Here's how the part is built. I have some questions about the finished solid (model axes, mm). Round coordinates to 2 decimals unless told otherwise and drop trailing zeros. Loops run counter-clockwise (first coordinate to the right, second up) from the corner with the lowest first, then second, coordinate; pieces in that order, holes last. Notation, with made-up numbers: M 83.25,18.25 L 117.25,18.25 A26 cw 117.25,40.25 Z; hole C -6.75,-25 d1. An arc over 180 degrees is marked long. Answer as a JSON object with one key per item and string values.
from build123d import *

# Parameters (mm, degrees)
SKETCH1_W           = 49
SKETCH1_H           = 33
SKETCH1_R           = 1.6
BOSS_EXTRUDE2_DEPTH = 3
FILLET1_R           = 2
SKETCH2_W           = 20
SKETCH2_H           = 27
CUT_EXTRUDE1_DEPTH  = 10


with BuildPart() as part:
    # Sketch1 → Boss-Extrude2 (new body)
    with BuildSketch(Plane.XY):
        with Locations((5.332147937, -0.241820768)):
            Rectangle(SKETCH1_W, SKETCH1_H)
        with Locations((-9.667852063, 9.758179232)):
            Circle(SKETCH1_R, mode=Mode.SUBTRACT)
        with Locations((20.332147937, 9.758179232)):
            Circle(SKETCH1_R, mode=Mode.SUBTRACT)
        with Locations((-9.667852063, -10.241820768)):
            Circle(SKETCH1_R, mode=Mode.SUBTRACT)
        with Locations((20.332147937, -10.241820768)):
            Circle(SKETCH1_R, mode=Mode.SUBTRACT)
    extrude(amount=BOSS_EXTRUDE2_DEPTH)

    # Fillet1
    fillet1_edges = [part.edges().sort_by_distance(p)[0] for p in [
        (-19.167852063, 16.258179232, 1.5),
        (29.832147937, 16.258179232, 1.5),
        (29.832147937, -16.741820768, 1.5),
        (-19.167852063, -16.741820768, 1.5),
    ]]
    fillet(fillet1_edges, radius=FILLET1_R)

    # Sketch2 → Cut-Extrude1 (cut)
    with BuildSketch(Plane.XY.offset(3)):
        with Locations((7.832147937, -0.241820768)):
            Rectangle(SKETCH2_W, SKETCH2_H)
    extrude(amount=-CUT_EXTRUDE1_DEPTH, mode=Mode.SUBTRACT)


solid = part.part
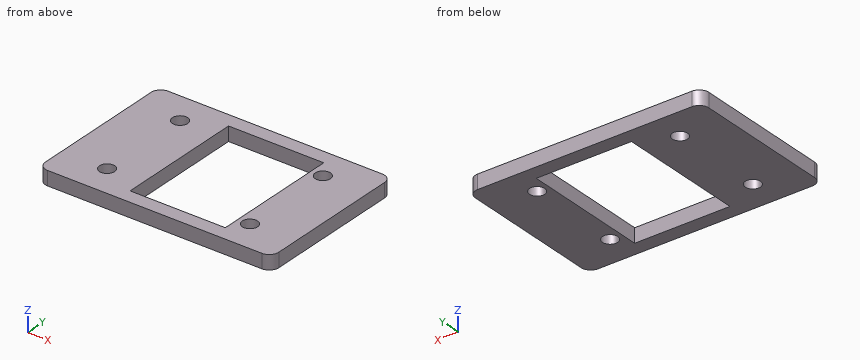
Item 1: I want a section at B-B, the plane y = -8. Please give me the cut outline in (x, z), then the cut area to 3 significant figures.
Resolved:
{"outline": "M -19.17,0 L -2.17,0 L -2.17,3 L -19.17,3 Z; M 17.83,0 L 29.83,0 L 29.83,3 L 17.83,3 Z", "area": "87.0 mm²"}
Item 2: I want a section at A-A, the plane x = -1.5. Please give me the cut outline in (y, z), then the cut area to 3 significant figures.
Resolved:
{"outline": "M -16.74,0 L -13.74,0 L -13.74,3 L -16.74,3 Z; M 13.26,0 L 16.26,0 L 16.26,3 L 13.26,3 Z", "area": "18.0 mm²"}
Item 3: I want a section at C-C, the plane y = 10.5. Please give me the cut outline in (x, z).
Resolved:
{"outline": "M -19.17,0 L -11.09,0 L -11.09,3 L -19.17,3 Z; M -8.25,0 L -2.17,0 L -2.17,3 L -8.25,3 Z; M 17.83,0 L 18.91,0 L 18.91,3 L 17.83,3 Z; M 21.75,0 L 29.83,0 L 29.83,3 L 21.75,3 Z"}
Item 4: I want a section at D-D, the plane z = 1.3. Please give me the cut outline in (x, y).
Resolved:
{"outline": "M -19.17,-14.74 A2 ccw -17.17,-16.74 L 27.83,-16.74 A2 ccw 29.83,-14.74 L 29.83,14.26 A2 ccw 27.83,16.26 L -17.17,16.26 A2 ccw -19.17,14.26 Z; hole C -9.67,-10.24 d3.2; hole C -9.67,9.76 d3.2; hole M -2.17,-13.74 L 17.83,-13.74 L 17.83,13.26 L -2.17,13.26 Z; hole C 20.33,-10.24 d3.2; hole C 20.33,9.76 d3.2"}
Item 5: Please list where these lines run through material, in increasing order: probe 1 along Y at (x, z) = (5.5, 2.7); probe 2 along X at (y, z) = (12.5, 2.6); probe 3 along Y at (x, z) = (21.5, 1.85). Write a range as from..to.
Resolved:
{"probe 1": "-16.74..-13.74, 13.26..16.26", "probe 2": "-19.17..-2.17, 17.83..29.83", "probe 3": "-16.74..-11.34, -9.15..8.66, 10.85..16.26"}
Item 6: I'm going to push a flat-ended pin straight in: pin 1 Ø3 at (x, y) = (-9.67, -10.24) entering from -Z. Where does the tip first touch, or does it pass through?
Resolved:
{"pin 1": "through"}
